from build123d import *

# Parameters (mm, degrees)
EXT_HEX_DEPTH = 1.905


with BuildPart() as part:
    # Sk_hex → Ext_hex (new body)
    with BuildSketch(Plane(origin=(0, 64.4906, 0), x_dir=(1, 0, 0), z_dir=(0, 1, 0))):
        Polygon((22.143692224, 0), (11.071846112, -19.177), (-11.071846112, -19.177), (-22.143692224, 0), (-11.071846112, 19.177), (11.071846112, 19.177), align=None)
    extrude(amount=EXT_HEX_DEPTH)

    # Sk_hex_bore → Cut_hex_bore (revolve, cut)
    with BuildSketch(Plane.XY, mode=Mode.PRIVATE) as cut_hex_bore_sk:
        with BuildLine():
            Line((0, 64.008), (12.97178, 64.008))
            Line((12.97178, 64.008), (12.97178, 64.4906))
            Line((12.97178, 64.4906), (15.45717, 66.19494))
            ThreePointArc((15.45717, 66.19494), (15.611327894, 66.297467411), (15.76832, 66.3956))
            Line((15.76832, 66.3956), (15.76832, 66.802))
            Line((15.76832, 66.802), (0, 66.802))
            Line((0, 66.802), (0, 64.008))
        make_face()
    revolve(cut_hex_bore_sk.sketch.rotate(Axis((0, -25.4, 0), (0, 1, 0)), 90), axis=Axis((0, -25.4, 0), (0, 1, 0)), mode=Mode.SUBTRACT)


solid = part.part
The listing builds one solid part. Answer for the finished solid, in the listing's coordinates (mm). Give positions to 0.01 mm unless a question says otherwise; leave off trailing zeros. Write each loop counter-clockwise with the first axis right and the second up, starting at its lowest first coordinate (ties: lowest second). Pieces come first, ordered by that corner, then holes.
1) Section B-B (x = 0) is taken. Write down the section's boundary in (y, z), and give its area (3 significant figures).
2) Section A-A (y = 65.7) is taken. Write down the section's boundary in (x, z), and give its area (3 significant figures).
3) Find the intervals of material crossed by L1, parallel to Z at x = 7.5, y = 66.35; L2, parallel to Z at x = -12, y = 66; L3, parallel to X at y = 64.6, z = 1, in increasing order.
Response:
1. outline: (64.49, -19.18) - (66.4, -19.18) - (66.4, -15.77) arc R6.55 ccw to (66.19, -15.46) - (64.49, -12.97) - close; (64.49, 12.97) - (66.19, 15.46) arc R6.55 ccw to (66.4, 15.77) - (66.4, 19.18) - (64.49, 19.18) - close
1. area: 18.3 mm2
2. outline: (-22.14, 0) - (-11.07, -19.18) - (11.07, -19.18) - (22.14, 0) - (11.07, 19.18) - (-11.07, 19.18) - close; hole circle Ø29.47 at (0, 0)
2. area: 592 mm2
3. L1: z = -19.18 to -13.79, 13.79 to 19.18
3. L2: z = -17.57 to -9.29, 9.29 to 17.57
3. L3: x = -21.57 to -13.09, 13.09 to 21.57
